```python
from build123d import *

# Parameters (mm, degrees)
CROQUIS1_W              = 25
CROQUIS1_H              = 25
SALIENTE_EXTRUIR1_DEPTH = 20
CROQUIS2_R              = 10
SALIENTE_EXTRUIR2_DEPTH = 10
CROQUIS3_R              = 9
CORTAR_EXTRUIR1_DEPTH   = 20
VACIADO2_OUTLINE_W      = 23
VACIADO2_OUTLINE_H      = 21
VACIADO2_DEPTH          = 9
VACIADO2_START          = 9
VACIADO2_2_OUTLINE_W    = 23
VACIADO2_2_OUTLINE_H    = 21
VACIADO2_2_OUTLINE_R    = 10
VACIADO2_2_DEPTH        = 10


# Read off the part's stored shape, not the designer's step: Vaciado2
with BuildPart() as part:
    # Croquis1 → Saliente-Extruir1 (new body)
    with BuildSketch(Plane(origin=(0, 0, 0), x_dir=(1, 0, 0), z_dir=(0, 1, 0))):
        Rectangle(CROQUIS1_W, CROQUIS1_H)
    extrude(amount=SALIENTE_EXTRUIR1_DEPTH)

    # Croquis2 → Saliente-Extruir2 (add)
    with BuildSketch(Plane(origin=(0, 20, 0), x_dir=(1, 0, 0), z_dir=(0, 1, 0))):
        with Locations(Location((0, 0, 0), (0, 0, 270))):
            Circle(CROQUIS2_R)
    extrude(amount=SALIENTE_EXTRUIR2_DEPTH)

    # Croquis3 → Cortar-Extruir1 (cut)
    with BuildSketch(Plane(origin=(0, 30, 0), x_dir=(1, 0, 0), z_dir=(0, 1, 0))):
        with Locations(Location((0, 0, 0), (0, 0, 270))):
            Circle(CROQUIS3_R)
    extrude(amount=-CORTAR_EXTRUIR1_DEPTH, mode=Mode.SUBTRACT)

    # Vaciado2 outline → Vaciado2 (cut)
    with BuildSketch(Plane(origin=(0, 0, 0), x_dir=(1, 0, 0), z_dir=(0, 1, 0))):
        Rectangle(VACIADO2_OUTLINE_W, VACIADO2_OUTLINE_H)
    extrude(amount=VACIADO2_DEPTH, mode=Mode.SUBTRACT)

    # Vaciado2 2 outline → Vaciado2 2 (cut)
    with BuildSketch(Plane(origin=(0, 0, 0), x_dir=(1, 0, 0), z_dir=(0, 1, 0)).offset(VACIADO2_START)):
        Rectangle(VACIADO2_2_OUTLINE_W, VACIADO2_2_OUTLINE_H)
        Circle(VACIADO2_2_OUTLINE_R, mode=Mode.SUBTRACT)
    extrude(amount=VACIADO2_2_DEPTH, mode=Mode.SUBTRACT)


solid = part.part
```
Model file for the job. Use its own axes, mm. A direction names the side the tool comes from. Round coordinates to 2 decimals unless told otherwise and drop trailing zeros. Loops run counter-clockwise (first coordinate to the right, second up) from the corner with the lowest first, then second, coordinate; pieces in that order, holes last. Notation, with made-up numbers: M 52.5,16 L 58.5,16 A36 ccw 58.5,52 Z; hole C -10.5,-25 d10. An arc over 180 degrees is marked long. Put each result on its own line as item: value. Start each with the question number.
Item 1: Drop flat-ended pins along their axis: P1, Ø1, axis at y = 21, z = 8.5, coming from the +X side; P2, Ø14.5, axis at x = 0, z = 0, coming from the -Y side; P3, Ø5.5, axis at x = 3, z = 2, coming from the +Y side. Give the stop position or say it passes through.
Item 2: Cut at A-A (y = 13.5). List the corners of the cut face in (x, z).
Item 3: Cut at C-C (y = 8.25). List the corners of the cut face in (x, z).
Item 4: Cut at B-B (x = 0). List the corners of the cut face in (y, z).
Item 5: 3-axis set-ups, long thin cutter, end or side, ignore diameter. For faces 1 (the face through (-10.4, 19, -0.1)), 2 (the face through (-1, 0, 11)), 3 (the face through (-9.76, 24.93, -2.17)): which of +Z, -Z, +X, -X, +Y, -Y reach the whole face in a straight line?
Item 6: Cut at D-D (z = 0). List the corners of the cut face in (x, y), then the cut area to 3 significant figures.
Item 7: Mould opens along X. For faces 4 (the face through (-12.5, 10, 0)), 5 (the face through (0, 9, 10.5)), 6 (the face through (0, 10, 12.5)) say: released by +X, released by -X, zero draft, split by the parting line, or undercut.
Item 8: Drill centre lines: line 1 along X through (y, z) = (18, 0); line 2 along Z through (x, y) = (7.75, 6.5); line 3 along Z through (x, y) = (3.5, 17.5). Where is each one in solid material? Low to high.
Answer block:
1. P1: x = 6
1. P2: y = 9
1. P3: y = 10
2. outline: M -12.5,-12.5 L 12.5,-12.5 L 12.5,12.5 L -12.5,12.5 Z; C 0,0 d20; hole M -11.5,-10.5 L 11.5,-10.5 L 11.5,10.5 L -11.5,10.5 Z; hole C 0,0 d18
3. outline: M -12.5,-12.5 L 12.5,-12.5 L 12.5,12.5 L -12.5,12.5 Z; hole M -11.5,-10.5 L 11.5,-10.5 L 11.5,10.5 L -11.5,10.5 Z
4. outline: M 0,-12.5 L 20,-12.5 L 20,-10 L 30,-10 L 30,-9 L 10,-9 L 10,9 L 30,9 L 30,10 L 20,10 L 20,12.5 L 0,12.5 L 0,10.5 L 19,10.5 L 19,10 L 9,10 L 9,-10 L 19,-10 L 19,-10.5 L 0,-10.5 Z
5. face 1: -Y
5. face 2: +Z, -Z, +X, -X, -Y
5. face 3: +Y
6. outline: M -12.5,0 L -11.5,0 L -11.5,19 L -10,19 L -10,9 L 10,9 L 10,19 L 11.5,19 L 11.5,0 L 12.5,0 L 12.5,20 L 10,20 L 10,30 L 9,30 L 9,10 L -9,10 L -9,30 L -10,30 L -10,20 L -12.5,20 Z
6. area: 103 mm2
7. face 4: released by -X
7. face 5: undercut
7. face 6: zero draft
8. line 1: -12.5 to -11.5, -10 to -9, 9 to 10, 11.5 to 12.5
8. line 2: -12.5 to -10.5, 10.5 to 12.5
8. line 3: -12.5 to -10.5, -9.37 to -8.29, 8.29 to 9.37, 10.5 to 12.5
